Verification items for this drawing (mm, ordinates from the low corner). A direction names the side the tool comes from. Give positions to 0.01 mm unless a question says otherwise; leave off trailing zeros. Order: outer loops, then holes, each group sorted by start corner. A loop starts at its lowest first (then second) coordinate and runs counter-clockwise, first axis right, second up.
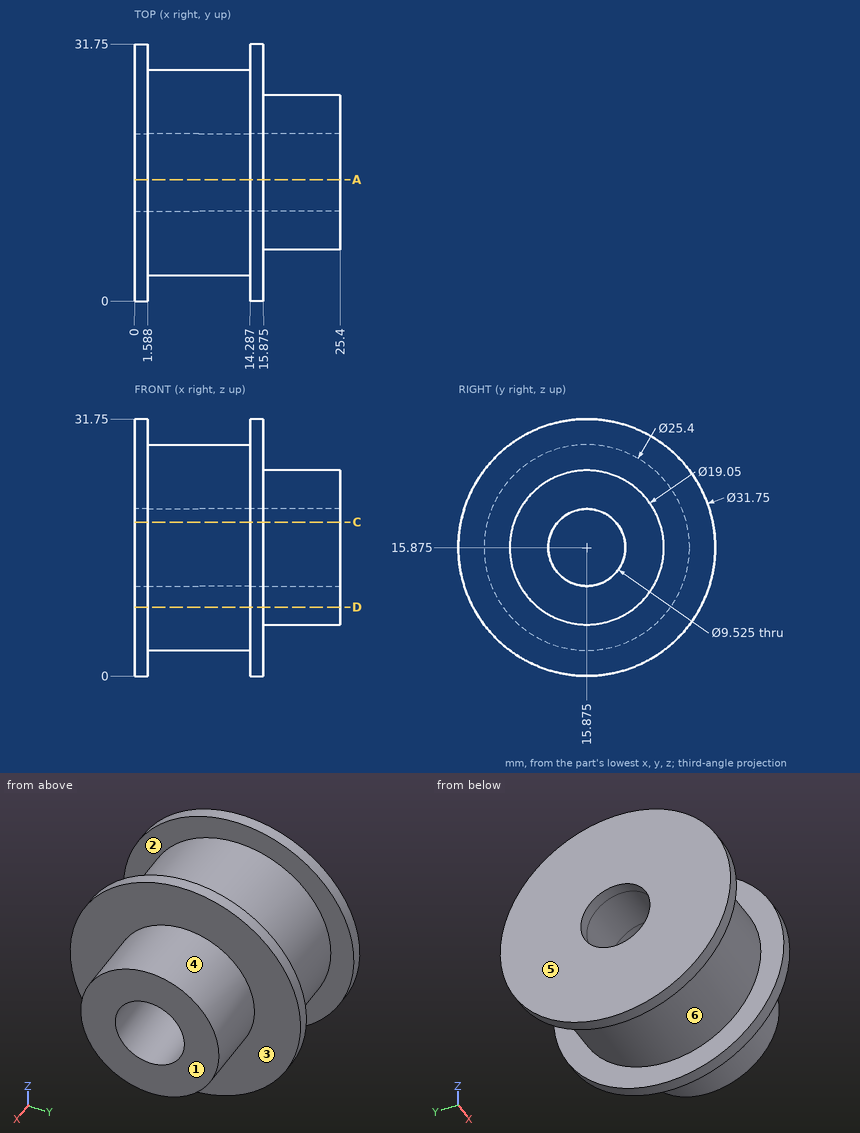
Q1. Cross-section at C-C, the plane z = 19. Record the boundary of the cut face in (x, y) (1 decimal), and give its area (3 significant figures).
Q2. Gauge pin test, flat ends, axial feed: P1, Ø1.5, axis at x = 17, z = 9.5, coming from the -Y side; P2, Ø4, axis at y = 26, z = 25.5, coming from the +X side (1 decimal); P3, Ø5, axis at x = 8, z = 13.5, coming from the -Y side (1 decimal); P4, Ø8.5, axis at y = 15.875, z = 15.875, coming from the -X side. Record the tip position at first contact, or that the pin passes through.
Q3. Thickness scan on L1, parallel to X at y = 24, z = 26 (1 decimal); L2, parallel to X at y = 6.5, z = 13 (1 decimal); L3, parallel to Y at x = 21.25, z = 19.5 (1 decimal). Record the ranges inside material, lowest first.
Q4. Release check for a two-part mould opening along X. For the marked faces 3, 4, 5 and 6 record: pulls with the +X half, pulls with the -X half, needs draft (parallel to the pull), parting line crosses it, or undercut.
Q5. Access from +Z, -Z, +X, -X, +Y, -Y to the whole of each face (thin tool, end or side, straight path). Record for the marked faces 1 and 2.
Q6. Cross-section at D-D, the plane z = 8.5. Record the boundary of the cut face in (x, y) (1 decimal).
Q7. Cross-section at A-A, the plane y = 15. Record the boundary of the cut face in (x, z) (1 decimal).
Answers follow:
1. outline: (0, 0.3) - (1.6, 0.3) - (1.6, 3.6) - (14.3, 3.6) - (14.3, 0.3) - (15.9, 0.3) - (15.9, 6.9) - (25.4, 6.9) - (25.4, 12.3) - (0, 12.3) - close; (0, 19.5) - (25.4, 19.5) - (25.4, 24.9) - (15.9, 24.9) - (15.9, 31.4) - (14.3, 31.4) - (14.3, 28.2) - (1.6, 28.2) - (1.6, 31.4) - (0, 31.4) - close
1. area: 400 mm2
2. P1: stops at y = 8.19
2. P2: stops at x = 15.9
2. P3: stops at y = 3.2
2. P4: passes through
3. L1: x = 0 to 1.6, 14.3 to 15.9
3. L2: x = 0 to 15.9
3. L3: y = 7.1 to 12.8, 19 to 24.7
4. face 3: pulls with the +X half
4. face 4: needs draft
4. face 5: pulls with the -X half
4. face 6: undercut
5. face 1: +Z, -Z, +X, +Y, -Y
5. face 2: none
6. outline: (0, 1.8) - (1.6, 1.8) - (1.6, 5.5) - (14.3, 5.5) - (14.3, 1.8) - (15.9, 1.8) - (15.9, 9.8) - (25.4, 9.8) - (25.4, 21.9) - (15.9, 21.9) - (15.9, 29.9) - (14.3, 29.9) - (14.3, 26.2) - (1.6, 26.2) - (1.6, 29.9) - (0, 29.9) - close
7. outline: (0, 0) - (1.6, 0) - (1.6, 3.2) - (14.3, 3.2) - (14.3, 0) - (15.9, 0) - (15.9, 6.4) - (25.4, 6.4) - (25.4, 11.2) - (0, 11.2) - close; (0, 20.6) - (25.4, 20.6) - (25.4, 25.4) - (15.9, 25.4) - (15.9, 31.7) - (14.3, 31.7) - (14.3, 28.5) - (1.6, 28.5) - (1.6, 31.7) - (0, 31.7) - close
